The drawing under review shows one solid part. Ordinate dimensions are in mm from its lowest x, y, z. Coordinates: 2 decimals unless noted, no trailing zeros. Loops run counter-clockwise (first coordinate to the right, second up) from the corner with the lowest first, then second, coordinate; pieces in that order, holes last. Notation, with made-up numbers: (39.25, -27.5) - (57.25, -27.5) arc R5 cw to (57.25, -20.5) - close; hole circle Ø10 at (-38.5, 65.5). An arc over 180 degrees is marked (long way). Use one line per item in the form item = value. Start each with the question number.
1. Add section C-C on z = 94. Give the boundary of the cut face in (x, y).
2. Add section B-B on z = 116. Give the boundary of the cut face in (x, y), and give its area (3 significant figures).
3. Add section D-D on x = 23. Give the boundary of the cut face in (y, z).
4. To check wall thickness, follow probe 1 along X at (y, z) = (5.25, 20); probe 2 along Z at (x, y) = (66.5, 6); probe 3 along X at (y, z) = (5.75, 77). State the ranges of each line that lie inside material, in increasing order.
5. Add section A-A on x = 40. Give the boundary of the cut face in (y, z).
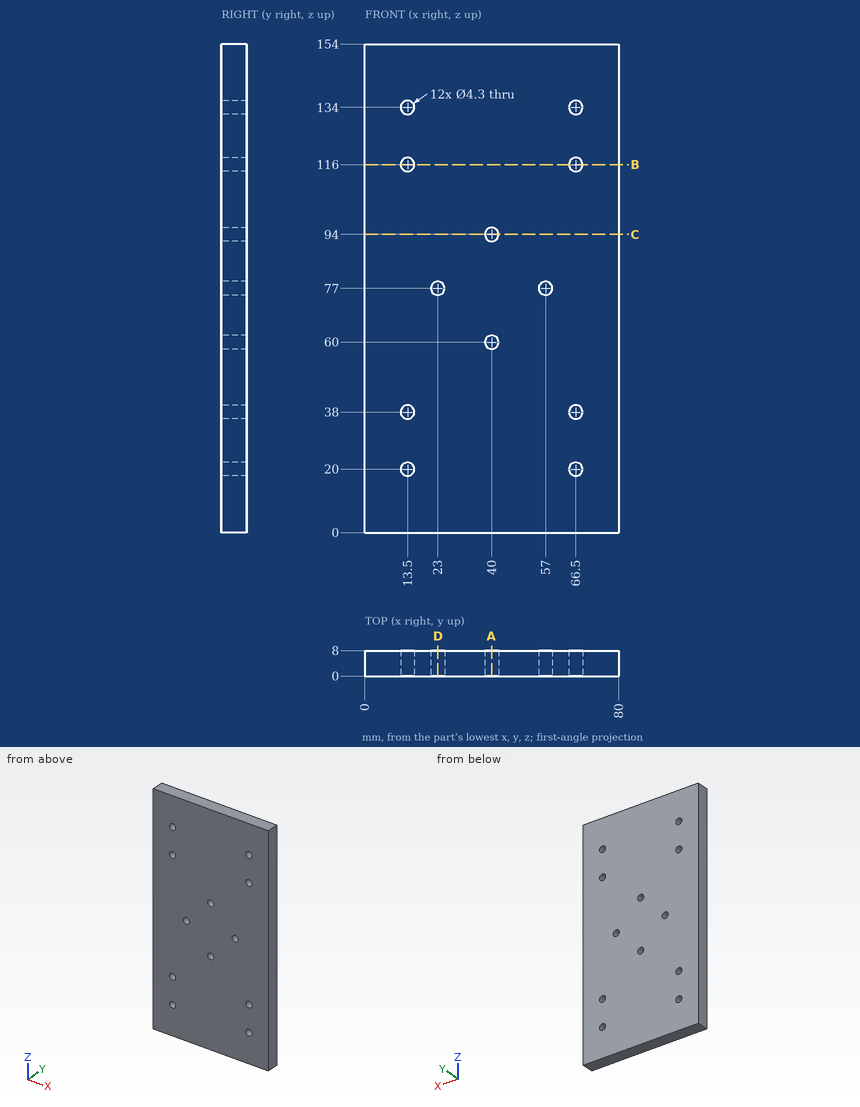
Conclusion:
q1.outline = (0, 0) - (37.85, 0) - (37.85, 8) - (0, 8) - close; (42.15, 0) - (80, 0) - (80, 8) - (42.15, 8) - close
q2.outline = (0, 0) - (11.35, 0) - (11.35, 8) - (0, 8) - close; (15.65, 0) - (64.35, 0) - (64.35, 8) - (15.65, 8) - close; (68.65, 0) - (80, 0) - (80, 8) - (68.65, 8) - close
q2.area = 571 mm^2
q3.outline = (0, 0) - (8, 0) - (8, 74.85) - (0, 74.85) - close; (0, 79.15) - (8, 79.15) - (8, 154) - (0, 154) - close
q4.probe_1 = 0 to 11.35, 15.65 to 64.35, 68.65 to 80
q4.probe_2 = 0 to 17.85, 22.15 to 35.85, 40.15 to 113.85, 118.15 to 131.85, 136.15 to 154
q4.probe_3 = 0 to 20.85, 25.15 to 54.85, 59.15 to 80
q5.outline = (0, 0) - (8, 0) - (8, 57.85) - (0, 57.85) - close; (0, 62.15) - (8, 62.15) - (8, 91.85) - (0, 91.85) - close; (0, 96.15) - (8, 96.15) - (8, 154) - (0, 154) - close
